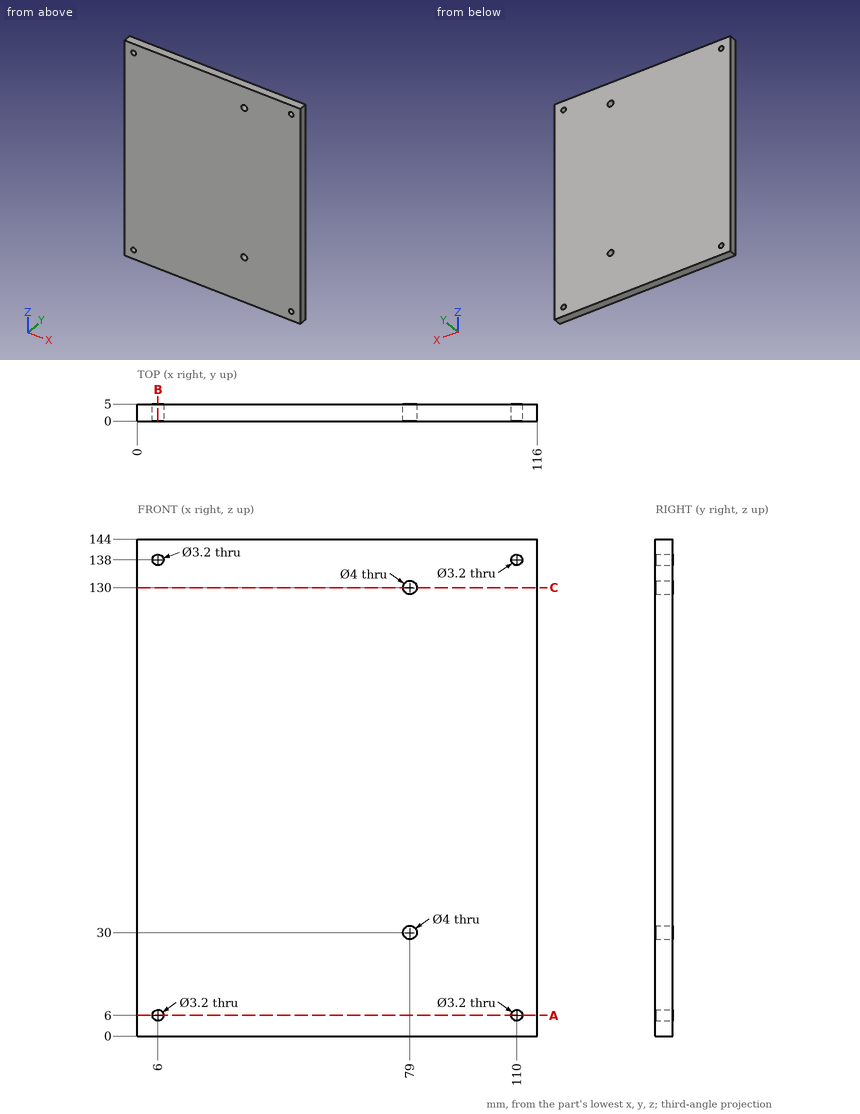
Here's the drawing with two shaded views (mm, measured from the low corner). I have some questions. Round coordinates to 2 decimals unless told otherwise and drop trailing zeros. Loops run counter-clockwise (first coordinate to the right, second up) from the corner with the lowest first, then second, coordinate; pieces in that order, holes last. Notation, with made-up numbers: M 11.5,-32.75 L 18.5,-32.75 A28 cw 18.5,-5.75 Z; hole C 75,10.5 d9. An arc over 180 degrees is marked long. Answer as a JSON object with one key per item and string values. Group by question number.
Q1. Please list where these lines run through material, in increasing order: L1, parallel to Z at x = 110, y = 1.4; L2, parallel to Z at x = 79, y = 1.2; L3, parallel to X at y = 2.75, z = 130.
Q2. Imagine slicing it at C-C, the plane z = 130. Please give me the cut outline in (x, y), then the cut area to 3 significant figures.
Q3. Imagine slicing it at A-A, the plane z = 6. Please give me the cut outline in (x, y), then the cut area to 3 significant figures.
Q4. Imagine slicing it at B-B, the plane x = 6. Please give me the cut outline in (y, z), then the cut area to 3 significant figures.
Findings:
{
 "1": {"L1": "z = 0 to 4.4, 7.6 to 136.4, 139.6 to 144", "L2": "z = 0 to 28, 32 to 128, 132 to 144", "L3": "x = 0 to 77, 81 to 116"},
 "2": {"outline": "M 0,0 L 77,0 L 77,5 L 0,5 Z; M 81,0 L 116,0 L 116,5 L 81,5 Z", "area": "560 mm2"},
 "3": {"outline": "M 0,0 L 4.4,0 L 4.4,5 L 0,5 Z; M 7.6,0 L 108.4,0 L 108.4,5 L 7.6,5 Z; M 111.6,0 L 116,0 L 116,5 L 111.6,5 Z", "area": "548 mm2"},
 "4": {"outline": "M 0,0 L 5,0 L 5,4.4 L 0,4.4 Z; M 0,7.6 L 5,7.6 L 5,136.4 L 0,136.4 Z; M 0,139.6 L 5,139.6 L 5,144 L 0,144 Z", "area": "688 mm2"}
}
